Input: part model. Units: mm. Frame: model coordinates. Face numbers are marked on the shaded views. A direction names the side the tool comes from. Give positions to 0.01 mm unless a question says otherwise; leave off trailing zeros. Write each loop counter-clockwise with the first axis right and the second up, starting at its lowest first coordinate (ties: lowest second). Pieces come first, ordered by that corner, then holes.
```python
from build123d import *
from OCP.BRepFilletAPI import BRepFilletAPI_MakeChamfer

# Parameters (mm, degrees)
BOSS_EXTRUDE1_DEPTH = 13
CUT_EXTRUDE1_REACH  = 19.09
SKETCH2_W           = 3.5
SKETCH2_H           = 3.5
CHAMFER3_SIZE       = 1
CHAMFER3_SIZE2      = 2.475086853
SKETCH4_R           = 2.2
CUT_EXTRUDE3_DEPTH  = 9
FILLET1_R           = 1
CHAMFER4_SIZE       = 0.5
FILLET2_R           = 2
FILLET3_R           = 0.5
CHAMFER5_SIZE       = 0.3
CHAMFER5_SIZE2      = 2.854309336


with BuildPart() as part:
    # Sketch1 → Boss-Extrude1 (new body)
    with BuildSketch(Plane.XY):
        Polygon((-2.782258065, -2.595897682), (-0.20192428, 1.104102318), (-0.20192428, 2.104102318), (9.517741935, 2.104102318), (9.517741935, -3.595897682), (-2.782258065, -3.595897682), align=None)
    extrude(amount=BOSS_EXTRUDE1_DEPTH)

    # Sketch2 → Cut-Extrude1 (cut, up to next)
    with BuildSketch(Plane(origin=(0, 2.104102318, 0), x_dir=(1, 0, 0), z_dir=(0, 1, 0)), mode=Mode.PRIVATE) as cut_extrude1_sk1:
        with Locations((5.467741935, -1.75)):
            Rectangle(SKETCH2_W, SKETCH2_H)
    cut_extrude1_tool1 = extrude(cut_extrude1_sk1.sketch, amount=-CUT_EXTRUDE1_REACH, mode=Mode.PRIVATE) & part.part
    # Sketch2 → Cut-Extrude1 (cut, up to next)
    with BuildSketch(Plane(origin=(0, 2.104102318, 0), x_dir=(1, 0, 0), z_dir=(0, 1, 0)), mode=Mode.PRIVATE) as cut_extrude1_sk2:
        with Locations((5.467741935, -11.25)):
            Rectangle(SKETCH2_W, SKETCH2_H)
    cut_extrude1_tool2 = extrude(cut_extrude1_sk2.sketch, amount=-CUT_EXTRUDE1_REACH, mode=Mode.PRIVATE) & part.part
    add(cut_extrude1_tool1.solids().sort_by_distance((5.467742, 2.104102, 1.75))[0], mode=Mode.SUBTRACT)
    add(cut_extrude1_tool2.solids().sort_by_distance((5.467742, 2.104102, 11.25))[0], mode=Mode.SUBTRACT)

    # Chamfer3: one chamfer whose edges measure the first distance from different faces: ONE call of the kernel's chamfer builder (chamfer() names one face for all edges)
    chamfer3_edges_1 = [part.edges().sort_by_distance(p)[0] for p in [
        (3.717741935, 2.104102318, 1.75),
        (3.717741935, 2.104102318, 11.25),
    ]]
    chamfer3_side_1 = [part.faces().sort_by_distance(p)[0] for p in [
        (4.46311444, 2.104102318, 6.5),
    ]]
    chamfer3_edges_2 = [part.edges().sort_by_distance(p)[0] for p in [
        (7.217741935, -3.595897682, 1.75),
        (7.217741935, -3.595897682, 11.25),
    ]]
    chamfer3_side_2 = [part.faces().sort_by_distance(p)[0] for p in [
        (2.987756707, -3.595897682, 6.5),
    ]]
    chamfer3 = BRepFilletAPI_MakeChamfer(part.part.solid().wrapped)
    for e in chamfer3_edges_1:
        chamfer3.Add(CHAMFER3_SIZE, CHAMFER3_SIZE2, e.wrapped, chamfer3_side_1[0].wrapped)  # the first distance lies on this face
    for e in chamfer3_edges_2:
        chamfer3.Add(CHAMFER3_SIZE, CHAMFER3_SIZE2, e.wrapped, chamfer3_side_2[0].wrapped)  # the first distance lies on this face
    add(Compound.cast(chamfer3.Shape()), mode=Mode.REPLACE)

    # Sketch4 → Cut-Extrude3 (cut)
    with BuildSketch(Plane(origin=(9.517741935, 0, 0), x_dir=(0, 0, -1), z_dir=(1, 0, 0))):
        with Locations(Location((-6.5, -0.745897682, 0), (0, 0, 90))):
            Circle(SKETCH4_R)
    extrude(amount=-CUT_EXTRUDE3_DEPTH, mode=Mode.SUBTRACT)

    # Fillet1
    fillet1_edges = [part.edges().sort_by_distance(p)[0] for p in [
        (-2.782258065, -2.595897682, 6.5),
        (-0.20192428, 1.104102318, 6.5),
    ]]
    fillet(fillet1_edges, radius=FILLET1_R)

    # Chamfer4
    chamfer4_edges = [part.edges().sort_by_distance(p)[0] for p in [
        (-0.20192428, 2.104102318, 6.5),
    ]]
    chamfer(chamfer4_edges, length=CHAMFER4_SIZE)

    # Fillet2
    fillet2_edges = [part.edges().sort_by_distance(p)[0] for p in [
        (3.717741935, -0.370984535, 11.25),
        (7.217741935, -1.120810828, 11.25),
        (7.217741935, -1.120810828, 1.75),
        (3.717741935, -0.370984535, 1.75),
    ]]
    fillet(fillet2_edges, radius=FILLET2_R)

    # Fillet3
    fillet3_edges = [part.edges().sort_by_distance(p)[0] for p in [
        (7.217741935, 2.104102318, 1.75),
        (3.717741935, -3.595897682, 1.75),
        (7.217741935, 2.104102318, 11.25),
        (3.717741935, -3.595897682, 11.25),
        (2.717741935, 2.104102318, 1.75),
        (2.717741935, 2.104102318, 11.25),
        (8.217741935, -3.595897682, 1.75),
        (8.217741935, -3.595897682, 11.25),
    ]]
    fillet(fillet3_edges, radius=FILLET3_R)

    # Chamfer5
    chamfer5_edges = [part.edges().sort_by_distance(p)[0] for p in [
        (9.517741935, -2.945897682, 6.5),
    ]]
    chamfer5_side = [part.faces().sort_by_distance(p)[0] for p in [
        (9.517741935, 1.962155145, 6.5),
    ]]
    chamfer(chamfer5_edges, length=CHAMFER5_SIZE, length2=CHAMFER5_SIZE2, reference=chamfer5_side[0])


solid = part.part
```
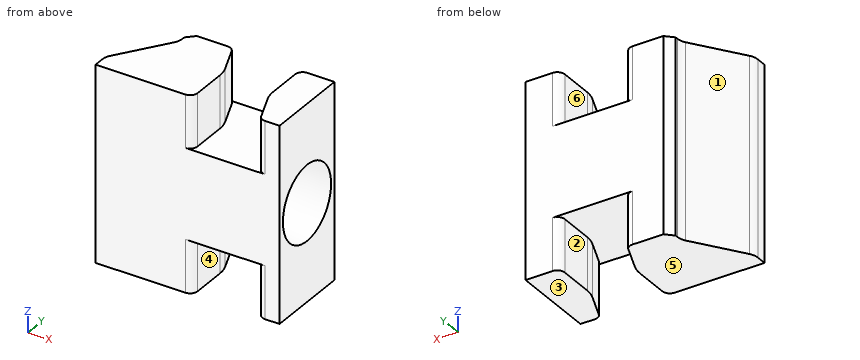
Item 1: Set-up query: the marked faces 4, 5 and 6. Return all of +Z, -Z, +X, -X, +Y, -Y with unobstructed straight access to the full face (end or side cutting, diameter ignored); none if empty.
Item 2: Mould query, pull axis X, two halves, no side actions, for the marked faces 1, 2 and 3. Classes: +X half, -X half, draft (parallel to the pull), parting line (faces both ways), or undercut.
Item 3: Section A-A (z = 6.5). Return loops of the section in (x, y).
Item 4: Section B-B (x = 4.25). Return loops of the section in (y, z), and give its area (3 significant figures).
Item 5: Ray query, line 1 (Z direction, x = 3, y = -0.8); line 2 (X direction, y = -0.8, z = 12.25); line 3 (Z direction, x = 2.5, y = -1.25). Return the intervals inside material, ascending.
Item 6: Pin query (flat end, axial travel): pin 1 (2 mm diameter, centred on y = -0.5, z = 6, fed in from +X); pin 2 (1.9 mm diameter, centred on y = 0.5, z = 12, fed in from -X); pin 3 (1.9 mm diameter, centred on y = 1, z = 1.5, fed in from -X). Return the tip coordinate at first contact, or that it passes through.
Item 7: Section C-C (z = 3.75). Return loops of the section in (x, y).
Solved:
1. face 4: -Z, +Y, -Y
1. face 5: -Z, +X, -X, +Y, -Y
1. face 6: +Z, +Y, -Y
2. face 1: -X half
2. face 2: undercut
2. face 3: draft
3. outline: (-2.78, -3.6) - (9.52, -3.6) - (9.52, -3.25) - (6.66, -2.95) - (0.52, -2.95) - (0.52, 1.45) - (6.66, 1.45) - (9.52, 1.75) - (9.52, 2.1) - (0.3, 2.1) - (-0.2, 1.6) - (-0.2, 1.42) arc R1 cw to (-0.38, 0.85) - (-2.6, -2.34) arc R1 ccw to (-2.78, -2.91) - close
4. outline: (-3.6, 3.5) - (2.1, 3.5) - (2.1, 9.5) - (-3.6, 9.5) - close; hole circle Ø4.4 at (-0.75, 6.5)
4. area: 19.0 mm2
5. line 1: z = 0 to 4.3, 8.7 to 13
5. line 2: x = -1.53 to 3.72, 7.22 to 9.52
5. line 3: z = 0 to 4.36, 8.64 to 13
6. pin 1: stops at x = 0.52
6. pin 2: stops at x = -1.29
6. pin 3: stops at x = -0.94
7. outline: (-2.78, -3.6) - (9.52, -3.6) - (9.52, 2.1) - (0.3, 2.1) - (-0.2, 1.6) - (-0.2, 1.42) arc R1 cw to (-0.38, 0.85) - (-2.6, -2.34) arc R1 ccw to (-2.78, -2.91) - close
